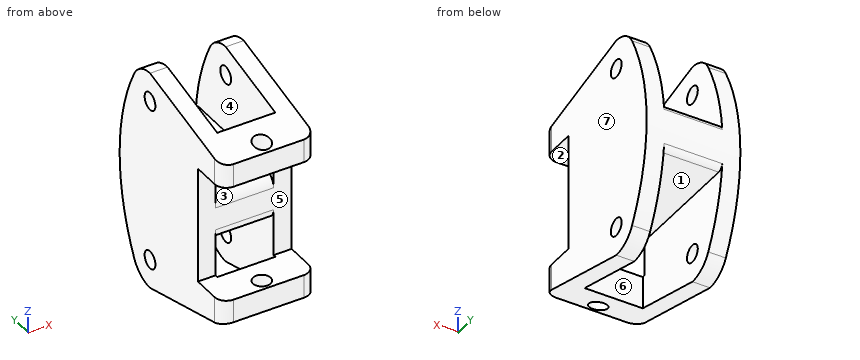
```python
from build123d import *

# Parameters (mm, degrees)
BOSS_EXTRUDE1_DEPTH = 16
SKETCH4_W           = 20
SKETCH4_H           = 6.652028381
CUT_EXTRUDE1_DEPTH  = 17
SKETCH5_R           = 1.5
CUT_EXTRUDE2_DEPTH  = 17
SKETCH6_W           = 9.919414232
SKETCH6_H           = 19.005976718
CUT_EXTRUDE3_DEPTH  = 23
FILLET3_R           = 2
FILLET6_R           = 1
SKETCH7_R           = 1.5
CUT_EXTRUDE4_DEPTH  = 40.7726311
FILLET7_R           = 2


with BuildPart() as part:
    # Sketch3 → Boss-Extrude1 (new body)
    with BuildSketch(Plane(origin=(0, 0, 0), x_dir=(0, 0, -1), z_dir=(1, 0, 0))):
        with BuildLine():
            Line((-14, 0), (14, 0))
            Line((14, 0), (19, 20))
            ThreePointArc((19, 20), (18.281744193, 22.581988897), (16.333333333, 24.422166387))
            ThreePointArc((16.333333333, 24.422166387), (0, 28.467001677), (-16.333333333, 24.422166387))
            ThreePointArc((-16.333333333, 24.422166387), (-18.281744193, 22.581988897), (-19, 20))
            Line((-19, 20), (-14, 0))
        make_face()
    extrude(amount=BOSS_EXTRUDE1_DEPTH)

    # Sketch4 → Cut-Extrude1 (cut, through all)
    with BuildSketch(Plane(origin=(16, 0, 0), x_dir=(0, 0, -1), z_dir=(1, 0, 0))):
        with Locations((0, 3.326014191)):
            Rectangle(SKETCH4_W, SKETCH4_H)
    extrude(amount=-CUT_EXTRUDE1_DEPTH, mode=Mode.SUBTRACT)

    # Sketch5 → Cut-Extrude2 (cut, through all)
    with BuildSketch(Plane.ZY):
        with Locations((-14.02107691, 20)):
            Circle(SKETCH5_R)
    cut_extrude2 = extrude(amount=-CUT_EXTRUDE2_DEPTH, mode=Mode.SUBTRACT)

    # Mirror3: Cut-Extrude2 across plane
    add(cut_extrude2.mirror(Plane.XY), mode=Mode.SUBTRACT)

    # Sketch6 → Cut-Extrude3 (cut)
    with BuildSketch(Plane(origin=(0, 29.164714895, 0), x_dir=(1, 0, 0), z_dir=(0, 1, 0))):
        with Locations((7.960322343, 13.441432697)):
            Rectangle(SKETCH6_W, SKETCH6_H)
    cut_extrude3 = extrude(amount=-CUT_EXTRUDE3_DEPTH, mode=Mode.SUBTRACT)

    # Mirror4: Cut-Extrude3 across plane
    add(cut_extrude3.mirror(Plane.XY), mode=Mode.SUBTRACT)

    # Fillet3
    fillet3_edges = [part.edges().sort_by_distance(p)[0] for p in [
        (7.960322343, 6.652028381, -3.938444338),
        (7.960322343, 6.652028381, 3.938444338),
    ]]
    fillet(fillet3_edges, radius=FILLET3_R)

    # Fillet6
    fillet6_edges = [part.edges().sort_by_distance(p)[0] for p in [
        (7.960322343, 28.244705112, -3.938444338),
        (7.960322343, 28.244705112, 3.938444338),
    ]]
    fillet(fillet6_edges, radius=FILLET6_R)

    # Sketch7 → Cut-Extrude4 (cut, through all)
    with BuildSketch(Plane.XY.offset(20.7726311)):
        with Locations((8.056637232, 2)):
            Circle(SKETCH7_R)
    extrude(amount=-CUT_EXTRUDE4_DEPTH, mode=Mode.SUBTRACT)

    # Fillet7
    fillet7_edges = [part.edges().sort_by_distance(p)[0] for p in [
        (0, 0, -12),
        (16, 0, -12),
        (16, 0, 12),
        (0, 0, 12),
    ]]
    fillet(fillet7_edges, radius=FILLET7_R)


solid = part.part
```
The listing builds one solid part. Answer for the finished solid, in the listing's coordinates (mm). Face numbers are marked on the shaded views. A direction names the side the tool comes from. Coordinates: 2 decimals unless noted, no trailing zeros. Loops run counter-clockwise (first coordinate to the right, second up) from the corner with the lowest first, then second, coordinate; pieces in that order, holes last. Notation, with made-up numbers: (-35.5, -36) -> (-30.5, -36) arc R23 ccw to (-30.5, -8) -> close; hole circle Ø1 at (5.25, 13). An arc over 180 degrees is marked (long way). Return JSON: item names as keys, results as strings. Group by question number.
(1) A cutting plane is placed at C-C on z = 8. Write down the section's boundary in (x, y), and give its area (3 significant figures).
(2) Which of the six approach directions +Z, -Z, +X, -X, +Y, -Y give full straight-line access (tool end or side, diameter ignored) to the marked faces 1, 2 and 3?
(3) Find the intervals of material crossed by probe 1 along X at (y, z) = (26, -11.5); probe 2 along Z at (x, y) = (3.5, 26.75); probe 3 along Z at (x, y) = (15, 5.75), in increasing order. Write a range as from..to.
(4) A cutting plane is placed at D-D on y = 26.5. Write down the section's boundary in (x, z).
(5) Given pin 1 Ø6 at (x, z) = (7.5, -12) entering from +Y; pin 2 Ø4 at (x, y) = (8.06, 2) entering from -Z; pin 3 Ø2.5 at (y, z) = (20, -14.02) entering from +X; pin 4 Ø3.5 at (x, y) = (4, 4.5) entering from +Z, each flat-ended and moving along its own axis, determine where each tip first touches the part or whether it passes through.
(6) A cutting plane is placed at B-B on y = 13. Write down the section's boundary in (x, z).
(7) A cutting plane is placed at A-A on x = 5. Write down the section's boundary in (y, z).
(8) Determine the mould class of the marked faces 4, 5, 6 and 7 for opening direction X: released by +X, released by -X, zero draft, split by the parting line, or undercut.
The answers:
{
 "1": {"outline": "(0, 6.65) -> (3, 6.65) -> (3, 27.54) -> (0, 27.54) -> close; (12.92, 6.65) -> (16, 6.65) -> (16, 27.54) -> (12.92, 27.54) -> close", "area": "127 mm^2"},
 "2": {"face 1": "-Z, +Y, -Y", "face 2": "+X, -X, -Y", "face 3": "+Z, -Y"},
 "3": {"probe 1": "x = 0..3, 12.92..16", "probe 2": "z = -3.94..3.94", "probe 3": "z = -15.44..-10, 10..15.44"},
 "4": {"outline": "(0, -11.57) -> (3, -11.57) -> (3, -3.94) -> (12.92, -3.94) -> (12.92, -11.57) -> (16, -11.57) -> (16, 11.57) -> (12.92, 11.57) -> (12.92, 3.94) -> (3, 3.94) -> (3, 11.57) -> (0, 11.57) -> close"},
 "5": {"pin 1": "stops at y = 6.16", "pin 2": "stops at z = -15", "pin 3": "passes through", "pin 4": "stops at z = 15.54"},
 "6": {"outline": "(0, -17.25) -> (3, -17.25) -> (3, -3.94) -> (12.92, -3.94) -> (12.92, -17.25) -> (16, -17.25) -> (16, 17.25) -> (12.92, 17.25) -> (12.92, 3.94) -> (3, 3.94) -> (3, 17.25) -> (0, 17.25) -> close"},
 "7": {"outline": "(0, -14) -> (6.16, -15.54) -> (6.16, -10) -> (0, -10) -> close; (0, 10) -> (6.16, 10) -> (6.16, 15.54) -> (0, 14) -> close; (6.65, -1.94) arc R2 ccw to (8.65, -3.94) -> (27.34, -3.94) arc R1 ccw to (28.34, -3.02) arc R35 ccw to (28.34, 3.02) arc R1 ccw to (27.34, 3.94) -> (8.65, 3.94) arc R2 ccw to (6.65, 1.94) -> close"},
 "8": {"face 4": "undercut", "face 5": "zero draft", "face 6": "undercut", "face 7": "released by +X"}
}
